Part model, mm, in its own coordinate system. Give positions to 0.01 mm unless a question says otherwise; leave off trailing zeros. Order: outer loops, then holes, each group sorted by start corner. A loop starts at its lowest first (then second) coordinate and runs counter-clockwise, first axis right, second up. Notation, with made-up numbers: M -38.5,54.5 L -20.5,54.5 A21 cw -20.5,93.5 Z; hole C 81,42 d9. An arc over 180 degrees is marked long. Answer as a JSON object with one key per item and string values.
from build123d import *

# Parameters (mm, degrees)
F1_DEPTH = 6


with BuildPart() as f1:
    # F0 (on Top) → F1 (new body)
    with BuildSketch(Plane.XY):
        with BuildLine():
            ThreePointArc((-782.8108229719, 316.071718416), (-782.9031509549, 316.304858246), (-783.026982617, 316.5229049295))
            ThreePointArc((-783.026982617, 316.5229049295), (-782.9094811402, 316.3018255077), (-782.8108229719, 316.071718416))
        make_face()
        with BuildLine():
            ThreePointArc((-783.7858049809, 313.886586525), (-784.7140567778, 313.7369427263), (-785.5911241746, 314.075760445))
            ThreePointArc((-785.5911241746, 314.075760445), (-786.452085755, 313.7016307347), (-787.3843295654, 313.8118548753))
            ThreePointArc((-787.3843295654, 313.8118548753), (-785.5833850086, 312.0137462238), (-783.7843305588, 313.8137459755))
            ThreePointArc((-783.7843305588, 313.8137459755), (-783.7846992021, 313.8501737107), (-783.7858049809, 313.886586525))
        make_face()
        with BuildLine():
            ThreePointArc((-787.3843295654, 313.8118548753), (-786.452085755, 313.7016307347), (-785.5911241746, 314.075760445))
            ThreePointArc((-785.5911241746, 314.075760445), (-786.1153495113, 314.6812963137), (-786.3249929012, 315.4543005447))
            ThreePointArc((-786.3249929012, 315.4543005447), (-787.0969927705, 314.7893755329), (-787.3843295654, 313.8118548753))
        make_face()
        with BuildLine():
            ThreePointArc((-786.3249929012, 315.4543005447), (-786.163887167, 316.2747079845), (-785.6495114244, 316.9338293848))
            ThreePointArc((-785.6495114244, 316.9338293848), (-788.2875683827, 316.3567553772), (-787.3843295654, 313.8118548753))
            ThreePointArc((-787.3843295654, 313.8118548753), (-787.0969927705, 314.7893755329), (-786.3249929012, 315.4543005447))
        make_face()
        with BuildLine():
            ThreePointArc((-785.6495114244, 316.9338293848), (-785.1089211657, 316.2968084324), (-784.9141692691, 315.4843398357))
            ThreePointArc((-784.9141692691, 315.4843398357), (-784.1140218759, 314.8521064028), (-783.7858049809, 313.886586525))
            ThreePointArc((-783.7858049809, 313.886586525), (-783.014317824, 314.5507170614), (-782.7264673233, 315.5271410942))
            ThreePointArc((-782.7264673233, 315.5271410942), (-782.7476812439, 315.8026770877), (-782.8108229719, 316.071718416))
            ThreePointArc((-782.8108229719, 316.071718416), (-782.9094811402, 316.3018255077), (-783.026982617, 316.5229049295))
            ThreePointArc((-783.026982617, 316.5229049295), (-784.2478248834, 317.3054432032), (-785.6495114244, 316.9338293848))
        make_face()
        with BuildLine():
            ThreePointArc((-784.9141692691, 315.4843398357), (-784.9141685241, 315.4833942858), (-784.9141682757, 315.4824487356))
            ThreePointArc((-784.9141682757, 315.4824487356), (-785.0922127612, 314.7018974503), (-785.5911241746, 314.075760445))
            ThreePointArc((-785.5911241746, 314.075760445), (-784.7140567778, 313.7369427263), (-783.7858049809, 313.886586525))
            ThreePointArc((-783.7858049809, 313.886586525), (-784.1140218759, 314.8521064028), (-784.9141692691, 315.4843398357))
        make_face()
        with BuildLine():
            ThreePointArc((-785.5911241746, 314.075760445), (-785.0922127612, 314.7018974503), (-784.9141682757, 315.4824487356))
            ThreePointArc((-784.9141682757, 315.4824487356), (-784.9141685241, 315.4833942858), (-784.9141692691, 315.4843398357))
            ThreePointArc((-784.9141692691, 315.4843398357), (-785.622647518, 315.6133380989), (-786.3249929012, 315.4543005447))
            ThreePointArc((-786.3249929012, 315.4543005447), (-786.1153495113, 314.6812963137), (-785.5911241746, 314.075760445))
        make_face()
        with BuildLine():
            ThreePointArc((-786.3249929012, 315.4543005447), (-785.622647518, 315.6133380989), (-784.9141692691, 315.4843398357))
            ThreePointArc((-784.9141692691, 315.4843398357), (-785.1089211657, 316.2968084324), (-785.6495114244, 316.9338293848))
            ThreePointArc((-785.6495114244, 316.9338293848), (-786.163887167, 316.2747079845), (-786.3249929012, 315.4543005447))
        make_face()
    extrude(amount=F1_DEPTH)


solid = f1.part
1. Cut at C-C on x = -783.9. Give the cut face in (y, z), plus the area to 3 significant figures.
Worked answers:
{"outline": "M 313.18,0 L 317.21,0 L 317.21,6 L 313.18,6 Z", "area": "24.2 mm^2"}
2. Two-plate mould, pull along X, no slides. Class faces 1 (the flat face through (-786, 315, 6)), 2 (the cylindrical face through (-788.27, 316.39, 2.96)): +X half, -X half, draft (parallel to the pull), parting line (faces both ways), or undercut.
Worked answers:
{"face 1": "draft", "face 2": "undercut"}
3. Pin check, flat tips, straight feed: P1, Ø3, axis at y = 312.5, z = 3, coming from the +X side; P2, Ø1.5, axis at y = 314, z = 4.5, coming from the +X side. Stop position of each tip, or through.
Worked answers:
{"P1": "stops at x = -783.57", "P2": "stops at x = -782.9"}
4. Cut at B-B on y = 312.95. Give the cut face in (x, z).
Worked answers:
{"outline": "M -787.16,0 L -784.01,0 L -784.01,6 L -787.16,6 Z"}
5. Probe line 1 along X through (y, z) = (313.3, 3); line 2 along Y through (x, z) = (-785.5, 2.95); line 3 along Y through (x, z) = (-783.45, 0.9). List the from-to ranges inside material, lowest first.
Worked answers:
{"line 1": "x = -787.31 to -783.86", "line 2": "y = 312.02 to 317.04", "line 3": "y = 314.08 to 316.97"}
